Verification items for the finished model (mm, model axes). Face numbers are marked on the shaded views. A direction names the side the tool comes from. Give positions to 0.01 mm unless a question says otherwise; leave off trailing zeros. Order: outer loops, then holes, each group sorted by start corner. A loop starts at its lowest first (then second) coordinate and runs counter-clockwise, first axis right, second up.
(1) Sectioned sample at D-D on z = -3.5. Record the cut outline in (x, y).
(2) Sectioned sample at A-A on x = 0. Record the cut outline in (y, z), plus the area to 3 significant figures.
(3) Mould release check, pull along Z, two halves, no side actions. Record for the marked faces 3, 4 and 5: pulls with the +Z half, pulls with the -Z half, needs draft (parallel to the pull), parting line crosses it, or undercut.
(4) Sectioned sample at B-B on z = 3.5. Record the cut outline in (x, y), plus the area to 3 significant figures.
(5) Gauge pin test, flat ends, axial feed: pin 1 (2 mm diameter, centred on x = -4.5, z = -3.5, fed in from -Y); pin 2 (2 mm diameter, centred on y = 16, z = -4.5, fed in from +X); pin 3 (3.5 mm diameter, centred on x = 0, z = 1, fed in from -Y). Record the tip position at first contact, or that the pin passes through.
(6) Access from +Z, -Z, +X, -X, +Y, -Y to the whole of each face (thin tool, end or side, straight path). Record for the marked faces 1 and 2.
(7) Scan lines: L1, parallel to Y at x = 2.75, z = -5; L2, parallel to X at y = 16.25, z = 1.25; L3, parallel to Z at x = -2, y = 10.5. Record each from-to range of solid material in increasing order.
(8) Sectioned sample at C-C on y = 5.25. Record the cut outline in (x, z), plus the area to 3 significant figures.
```python
from build123d import *

# Parameters (mm, degrees)
SKETCH5_R          = 3.1
CUT_EXTRUDE1_DEPTH = 23.649503306


with BuildPart() as part:
    # Sketch4 → Revolve1 (revolve)
    with BuildSketch(Plane(origin=(0, 0, 0), x_dir=(0, 0, -1), z_dir=(1, 0, 0)), mode=Mode.PRIVATE) as revolve1_sk:
        Polygon((-4.5, 2.5), (-5, 2.5), (-5, 7.5), (-6, 7.5), (-6, 21), (0, 21), (0, 0), (-4.5, 0), align=None)
    revolve(revolve1_sk.sketch.rotate(Axis((0, -43.514912226, 0), (0, 1, 0)), 180), axis=Axis((0, -43.514912226, 0), (0, 1, 0)))

    # Sketch5 → Cut-Extrude1 (cut, through all)
    with BuildSketch(Plane.XZ):
        with Locations(Location((0, 1, 0), (0, 0, 270))):
            Circle(SKETCH5_R)
    extrude(amount=-CUT_EXTRUDE1_DEPTH, mode=Mode.SUBTRACT)


solid = part.part
```
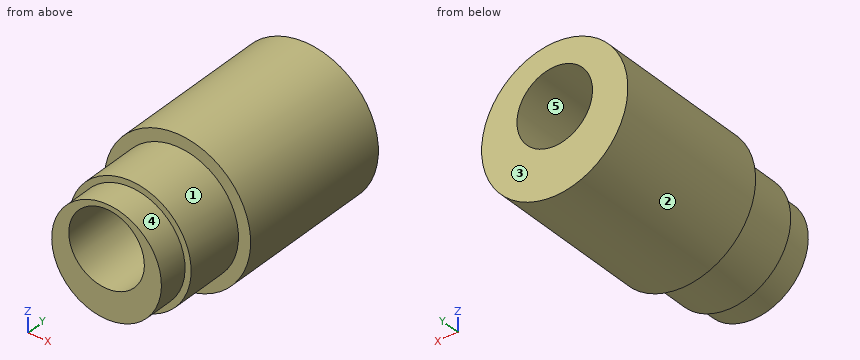
Ans:
1. outline: (-4.87, 7.5) - (-3.57, 7.5) - (-3.57, 2.5) - (-2.83, 2.5) - (-2.83, 0) - (2.83, 0) - (2.83, 2.5) - (3.57, 2.5) - (3.57, 7.5) - (4.87, 7.5) - (4.87, 21) - (-4.87, 21) - close
2. outline: (0, -4.5) - (2.5, -4.5) - (2.5, -5) - (7.5, -5) - (7.5, -6) - (21, -6) - (21, -2.1) - (0, -2.1) - close; (0, 4.1) - (21, 4.1) - (21, 6) - (7.5, 6) - (7.5, 5) - (2.5, 5) - (2.5, 4.5) - (0, 4.5) - close
2. area: 104 mm2
3. face 3: needs draft
3. face 4: parting line crosses it
3. face 5: undercut
4. outline: (-4.87, 7.5) - (-3.57, 7.5) - (-3.57, 2.5) - (-2.83, 2.5) - (-2.83, 0) - (-1.83, 0) - (-1.83, 21) - (-4.87, 21) - close; (1.83, 0) - (2.83, 0) - (2.83, 2.5) - (3.57, 2.5) - (3.57, 7.5) - (4.87, 7.5) - (4.87, 21) - (1.83, 21) - close
4. area: 104 mm2
5. pin 1: stops at y = 2.5
5. pin 2: stops at x = 4.87
5. pin 3: passes through
6. face 1: -Y
6. face 2: +Y, -Y
7. L1: y = 7.5 to 21
7. L2: x = -5.87 to -3.09, 3.09 to 5.87
7. L3: z = -5.66 to -1.37, 3.37 to 5.66
8. outline: circle Ø10 at (0, 0); hole circle Ø6.2 at (0, 1)
8. area: 48.3 mm2
